```python
from build123d import *

# Parameters (mm, degrees)
SKETCH_1_W          = 130
SKETCH_1_H          = 260
EXTRUDE_1_DEPTH     = 3
SKETCH_2_R          = 1.65
SKETCH_2_R_2        = 1.6
SKETCH_2_R_3        = 1.605
CUT_EXTRUDE_1_DEPTH = 3
SKETCH_3_W          = 50
SKETCH_3_H          = 50
CUT_EXTRUDE_2_DEPTH = 10
FILLET_1_R          = 15
CUT_EXTRUDE_4_DEPTH = 10


with BuildPart() as part:
    # 草图1 → 凸台-拉伸1 (new body)
    with BuildSketch(Plane.XY):
        with Locations((65, 130)):
            Rectangle(SKETCH_1_W, SKETCH_1_H)
    extrude(amount=EXTRUDE_1_DEPTH)

    # 草图2 → 切除-拉伸1 (cut)
    with BuildSketch(Plane.XY.offset(3)):
        with Locations((120, 10)):
            Circle(SKETCH_2_R)
        with Locations((10, 10)):
            Circle(SKETCH_2_R)
        with Locations(Location((10, 250, 0), (0, 0, 180))):
            Circle(SKETCH_2_R)
        with Locations(Location((120, 250, 0), (0, 0, 180))):
            Circle(SKETCH_2_R)
        with Locations((120, 130)):
            Circle(SKETCH_2_R_2)
        with Locations((10, 130)):
            Circle(SKETCH_2_R_3)
    extrude(amount=-CUT_EXTRUDE_1_DEPTH, mode=Mode.SUBTRACT)

    # 草图3 → 切除-拉伸2 (cut)
    with BuildSketch(Plane(origin=(0, 0, 0), x_dir=(-1, 0, 0), z_dir=(0, 0, -1))):
        with Locations((-65, 180)):
            Rectangle(SKETCH_3_W, SKETCH_3_H)
    extrude(amount=-CUT_EXTRUDE_2_DEPTH, mode=Mode.SUBTRACT)

    # 圆角1
    fillet_1_edges = [part.edges().sort_by_distance(p)[0] for p in [
        (0, 0, 1.5),
        (130, 0, 1.5),
        (130, 260, 1.5),
        (0, 260, 1.5),
    ]]
    fillet(fillet_1_edges, radius=FILLET_1_R)

    # 草图4 → 切除-拉伸4 (cut)
    with BuildSketch(Plane(origin=(0, 0, 0), x_dir=(-1, 0, 0), z_dir=(0, 0, -1))):
        with BuildLine():
            Line((-90, 12), (-40, 12))
            ThreePointArc((-40, 12), (-38, 10), (-40, 8))
            Line((-40, 8), (-90, 8))
            ThreePointArc((-90, 8), (-92, 10), (-90, 12))
        make_face()
        with BuildLine():
            Line((-90, 27), (-40, 27))
            ThreePointArc((-40, 27), (-38, 25), (-40, 23))
            Line((-40, 23), (-90, 23))
            ThreePointArc((-90, 23), (-92, 25), (-90, 27))
        make_face()
        with BuildLine():
            Line((-90, 42), (-40, 42))
            ThreePointArc((-40, 42), (-38, 40), (-40, 38))
            Line((-40, 38), (-90, 38))
            ThreePointArc((-90, 38), (-92, 40), (-90, 42))
        make_face()
        with BuildLine():
            Line((-90, 57), (-40, 57))
            ThreePointArc((-40, 57), (-38, 55), (-40, 53))
            Line((-40, 53), (-90, 53))
            ThreePointArc((-90, 53), (-92, 55), (-90, 57))
        make_face()
        with BuildLine():
            Line((-90, 72), (-40, 72))
            ThreePointArc((-40, 72), (-38, 70), (-40, 68))
            Line((-40, 68), (-90, 68))
            ThreePointArc((-90, 68), (-92, 70), (-90, 72))
        make_face()
        with BuildLine():
            Line((-90, 87), (-40, 87))
            ThreePointArc((-40, 87), (-38, 85), (-40, 83))
            Line((-40, 83), (-90, 83))
            ThreePointArc((-90, 83), (-92, 85), (-90, 87))
        make_face()
        with BuildLine():
            Line((-90, 102), (-40, 102))
            ThreePointArc((-40, 102), (-38, 100), (-40, 98))
            Line((-40, 98), (-90, 98))
            ThreePointArc((-90, 98), (-92, 100), (-90, 102))
        make_face()
        with BuildLine():
            Line((-90, 117), (-40, 117))
            ThreePointArc((-40, 117), (-38, 115), (-40, 113))
            Line((-40, 113), (-90, 113))
            ThreePointArc((-90, 113), (-92, 115), (-90, 117))
        make_face()
        with BuildLine():
            Line((-90, 132), (-40, 132))
            ThreePointArc((-40, 132), (-38, 130), (-40, 128))
            Line((-40, 128), (-90, 128))
            ThreePointArc((-90, 128), (-92, 130), (-90, 132))
        make_face()
        with BuildLine():
            Line((-90, 147), (-40, 147))
            ThreePointArc((-40, 147), (-38, 145), (-40, 143))
            Line((-40, 143), (-90, 143))
            ThreePointArc((-90, 143), (-92, 145), (-90, 147))
        make_face()
        with BuildLine():
            Line((-90, 222), (-40, 222))
            ThreePointArc((-40, 222), (-38, 220), (-40, 218))
            Line((-40, 218), (-90, 218))
            ThreePointArc((-90, 218), (-92, 220), (-90, 222))
        make_face()
        with BuildLine():
            Line((-90, 237), (-40, 237))
            ThreePointArc((-40, 237), (-38, 235), (-40, 233))
            Line((-40, 233), (-90, 233))
            ThreePointArc((-90, 233), (-92, 235), (-90, 237))
        make_face()
        with BuildLine():
            Line((-90, 252), (-40, 252))
            ThreePointArc((-40, 252), (-38, 250), (-40, 248))
            Line((-40, 248), (-90, 248))
            ThreePointArc((-90, 248), (-92, 250), (-90, 252))
        make_face()
    extrude(amount=-CUT_EXTRUDE_4_DEPTH, mode=Mode.SUBTRACT)


solid = part.part
```
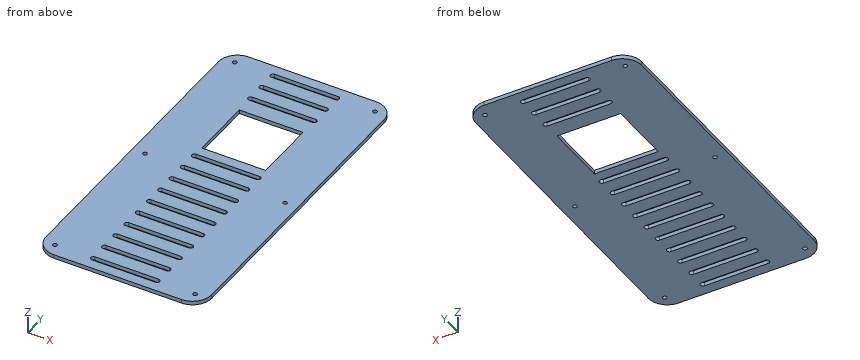
CAD build for the part. Positions are in the model's coordinates, mm. Round coordinates to 2 decimals unless told otherwise and drop trailing zeros. Order: outer loops, then holes, each group sorted by start corner. A loop starts at its lowest first (then second) coordinate and runs counter-clockwise, first axis right, second up.
Q1. Slice it at B-B (z = 0.6). State how many separate pieces and enclosed holes the cut face has, and give its area (3 significant figures).
Q2. Slice it at A-A (y = 201). Write the cut outline in (x, z).
Q3. Wall check: L1, parallel to X at y = 130, z = 0.7 (3 decimals); L2, parallel to X at y = 55, z = 2.15; L3, parallel to Y at x = 120, z = 0.7. Give the ranges that are in metal, low to high.
Results below:
1. separate pieces: 1
1. enclosed holes: 20
1. area: 28,300 mm2
2. outline: (0, 0) - (40, 0) - (40, 3) - (0, 3) - close; (90, 0) - (130, 0) - (130, 3) - (90, 3) - close
3. L1: x = 0 to 8.395, 11.605 to 38, 92 to 118.4, 121.6 to 130
3. L2: x = 0 to 38, 92 to 130
3. L3: y = 0.86 to 8.35, 11.65 to 128.4, 131.6 to 248.35, 251.65 to 259.14
